Drawing for the job (mm, zero at the part's lowest x, y, z). A direction names the side the tool comes from. Coordinates: 2 decimals unless noted, no trailing zeros. Order: outer loops, then holes, each group sorted by start corner. A loop starts at its lowest first (then second) coordinate and runs counter-clockwise, first axis right, second up. Notation, with made-up numbers: (4, -31.75) -> (23, -31.75) arc R9 ccw to (23, -25.75) -> close; hole circle Ø11 at (-14, 47). An arc over 180 degrees is marked (long way). Write each question's results on one line, items separated by ' | '.
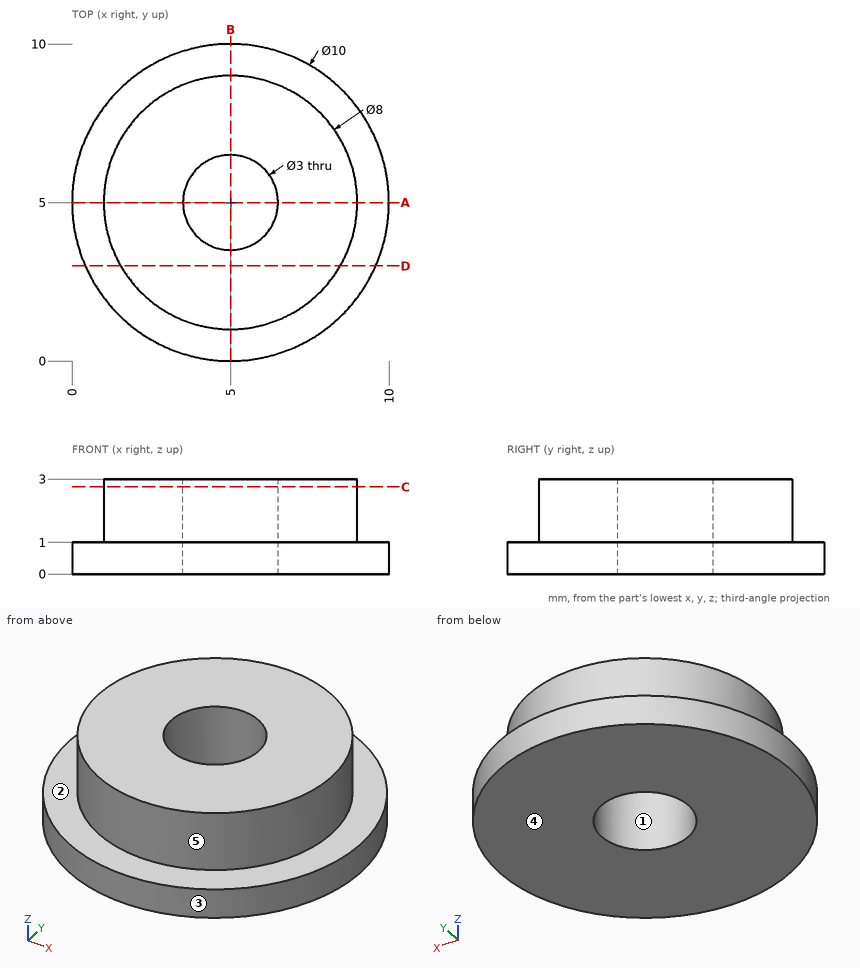
Item 1: Slice it at D-D, the plane y = 3. List the corners of the cut face in (x, z).
Answer:
outline: (0.42, 0) -> (9.58, 0) -> (9.58, 1) -> (8.46, 1) -> (8.46, 3) -> (1.54, 3) -> (1.54, 1) -> (0.42, 1) -> close
Item 2: Drill centre lines: line 1 (Z direction, x = 7.75, y = 8.5); line 2 (Y direction, x = 5, z = 1.75); line 3 (Y direction, x = 3.75, z = 0.8). Where is each one in solid material? Low to high. Write a range as from..to.
Answer:
line 1: z = 0..1 | line 2: y = 1..3.5, 6.5..9 | line 3: y = 0.16..4.17, 5.83..9.84
Item 3: Tool access for the marked faces 4 and 5: list every direction of +Z, -Z, +X, -X, +Y, -Y with a clear straight run to the whole face (end or side of a thin tool).
Answer:
face 4: -Z, +X, -X, +Y, -Y | face 5: +Z
Item 4: Pull direction Y, two halves, no side cores. Call the marked faces 1, 2 and 3: released by +Y, released by -Y, zero draft, split by the parting line, or undercut.
Answer:
face 1: undercut | face 2: zero draft | face 3: split by the parting line
Item 5: Slice it at C-C, the plane z = 2.75. List the corners of the cut face in (x, y), and give its area (3 significant figures).
Answer:
outline: circle Ø8 at (5, 5); hole circle Ø3 at (5, 5) | area: 43.2 mm^2
Item 6: Slice it at A-A, the plane y = 5. List the corners of the cut face in (x, z), and give its area (3 significant figures).
Answer:
outline: (0, 0) -> (3.5, 0) -> (3.5, 3) -> (1, 3) -> (1, 1) -> (0, 1) -> close; (6.5, 0) -> (10, 0) -> (10, 1) -> (9, 1) -> (9, 3) -> (6.5, 3) -> close | area: 17.0 mm^2
